from build123d import *

# Parameters (mm, degrees)
SKETCH2_R           = 2.25
BOSS_EXTRUDE1_DEPTH = 8
CUT_EXTRUDE1_REACH  = 25.345
SKETCH3_R           = 2.5


with BuildPart() as part:
    # Sketch2 → Boss-Extrude1 (new body)
    with BuildSketch(Plane.XY):
        Polygon((-8, 9), (8, 9), (10, 7), (10, -7), (8, -9), (-8, -9), (-10, -7), (-10, 7), align=None)
        with Locations((-6, 5)):
            Circle(SKETCH2_R, mode=Mode.SUBTRACT)
        with Locations((-6, -5)):
            Circle(SKETCH2_R, mode=Mode.SUBTRACT)
        with Locations((6, 5)):
            Circle(SKETCH2_R, mode=Mode.SUBTRACT)
        with Locations((6, -5)):
            Circle(SKETCH2_R, mode=Mode.SUBTRACT)
    extrude(amount=BOSS_EXTRUDE1_DEPTH)

    # Sketch3 → Cut-Extrude1 (cut, up to next)
    with BuildSketch(Plane(origin=(10, 0, 0), x_dir=(0, 0, -1), z_dir=(1, 0, 0)), mode=Mode.PRIVATE) as cut_extrude1_sk1:
        with Locations((-8.25, 0)):
            Circle(SKETCH3_R)
    cut_extrude1_tool1 = extrude(cut_extrude1_sk1.sketch, amount=-CUT_EXTRUDE1_REACH, mode=Mode.PRIVATE) & part.part
    add(cut_extrude1_tool1.solids().sort_by_distance((10, 0, 8.25))[0], mode=Mode.SUBTRACT)


solid = part.part
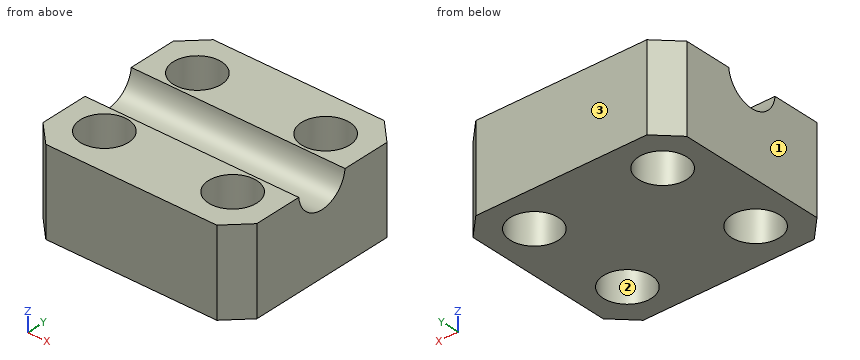
Can you work these out from the model? Positions are in its coordinate system, mm. Face numbers are marked on the shaded views. Coordinates: 2 decimals unless noted, no trailing zeros. Order: outer loops, then holes, each group sorted by start corner. A loop starts at its lowest first (then second) coordinate and runs counter-clockwise, first axis right, second up. Notation, with made-up numbers: M 53,46 L 65,46 A7 ccw 65,53 Z; hole C 35,40.25 d1. An arc over 180 degrees is marked long. Write item = value, one per line.
(1) If we mould it in two halves opening along X, with no side actions, what happens to the marked faces 1, 2 and 3? For each: pulls with the +X half, pulls with the -X half, needs draft (parallel to the pull), parting line crosses it, or undercut.
Results are:
face_1 = pulls with the -X half
face_2 = undercut
face_3 = needs draft
(2) Suppose I cut it at D-D on z = 7.25. Please give me the cut outline in (x, y), plus the area to 3 significant figures.
Results are:
outline = M -10,-7 L -8,-9 L 8,-9 L 10,-7 L 10,-2.29 L -10,-2.29 Z; M -10,2.29 L 10,2.29 L 10,7 L 8,9 L -8,9 L -10,7 Z; hole C -6,-5 d4.5; hole C -6,5 d4.5; hole C 6,-5 d4.5; hole C 6,5 d4.5
area = 197 mm2
(3) Suppose I cut it at B-B on z = 1.5. Please give me the cut outline in (x, y).
Results are:
outline = M -10,-7 L -8,-9 L 8,-9 L 10,-7 L 10,7 L 8,9 L -8,9 L -10,7 Z; hole C -6,-5 d4.5; hole C -6,5 d4.5; hole C 6,-5 d4.5; hole C 6,5 d4.5
(4) Suppose I cut it at A-A on x = -6. Please give me the cut outline in (y, z), plus the area to 3 significant figures.
Results are:
outline = M -9,0 L -7.25,0 L -7.25,8 L -9,8 Z; M -2.75,0 L 2.75,0 L 2.75,8 L 2.49,8 A2.5 cw -2.49,8 L -2.75,8 Z; M 7.25,0 L 9,0 L 9,8 L 7.25,8 Z
area = 63.4 mm2
(5) Suppose I cut it at C-C on y = 5. Please give me the cut outline in (x, z), plus the area to 3 significant figures.
Results are:
outline = M -10,0 L -8.25,0 L -8.25,8 L -10,8 Z; M -3.75,0 L 3.75,0 L 3.75,8 L -3.75,8 Z; M 8.25,0 L 10,0 L 10,8 L 8.25,8 Z
area = 88.0 mm2
(6) I need wall thicknesses on line 1 along Y through (x, z) = (6, 2.75); line 2 along Y through (x, z) = (-5.5, 7.5); line 3 along X through (y, z) = (-5.5, 2.25). Which ranges of each line are inside material? Lowest first, please. Write a range as [from, to].
Results are:
line_1 = [-9, -7.25], [-2.75, 2.75], [7.25, 9]
line_2 = [-9, -7.19], [-2.81, -2.38], [2.38, 2.81], [7.19, 9]
line_3 = [-10, -8.19], [-3.81, 3.81], [8.19, 10]
